The listing builds one solid part. Answer for the finished solid, in the listing's coordinates (mm). Face numbers are marked on the shaded views. A direction names the side the tool comes from. Round coordinates to 2 decimals unless told otherwise and drop trailing zeros. Loops run counter-clockwise (first coordinate to the right, second up) from the corner with the lowest first, then second, coordinate; pieces in that order, holes last. Notation, with made-up numbers: M 56.25,82 L 61.25,82 A35 cw 61.25,121 Z; hole C -12,-17 d6. An arc over 180 degrees is marked long. Answer as a JSON object with one key per item and string values.
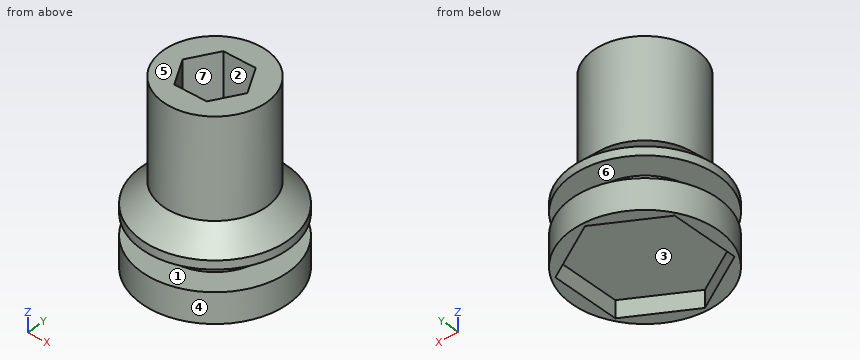
```python
from build123d import *

# Parameters (mm, degrees)
F0_R        = 8.5
F1_DEPTH    = 11
F3_DEPTH    = 2
F5_R        = 8.5
F5_R_2      = 5.5
F6_DEPTH    = 2.5
F7_R        = 6
F8_DEPTH    = 10
F9_S5_R     = 6
F9_T6_DEPTH = 14
F11_DEPTH   = 12


# Not quite as in the source:
# - a fillet or chamfer that OpenCascade refuses, or shapes differently, is made with other operations: its cross-section is extruded or revolved along the edge and cut away or added


with BuildPart() as f1:
    # F0 (on Top) → F1 (new body)
    with BuildSketch(Plane.XY):
        Circle(F0_R)
    extrude(amount=F1_DEPTH)

    # F2 (on face) → F3 (cut)
    with BuildSketch(Plane(origin=(0, 0, 0), x_dir=(1, 0, 0), z_dir=(0, 0, -1))):
        Polygon((7, 4.0414518843), (0, 8.0829037687), (-7, 4.0414518843), (-7, -4.0414518843), (0, -8.0829037687), (7, -4.0414518843), align=None)
    extrude(amount=-F3_DEPTH, mode=Mode.SUBTRACT)

    # F5 (on offset) → F6 (cut)
    with BuildSketch(Plane(origin=(0, 0, 3.5), x_dir=(1, 0, 0), z_dir=(0, 0, -1))):
        Circle(F5_R)
        Circle(F5_R_2, mode=Mode.SUBTRACT)
    extrude(amount=-F6_DEPTH, mode=Mode.SUBTRACT)

    # F7 (on face) → F8 (join)
    with BuildSketch(Plane.XY.offset(11)):
        Circle(F7_R)
    extrude(amount=F8_DEPTH)

    # F9: chamfer of 4 on 1 edges, made by hand


with BuildPart() as f9_tool2:
    # F9_s3 → F9_t4 (revolve)
    with BuildSketch(Plane.XZ):
        Polygon((8.5, 7), (4.5, 11), (8.5, 11), align=None)
    revolve(axis=Axis((0, 0, 11), (0, 0, 1)))

    # F9_s5 → F9_t6 (cut, symmetric)
    with BuildSketch(Plane.XY.offset(9)):
        Circle(F9_S5_R)
    extrude(amount=F9_T6_DEPTH, both=True, mode=Mode.SUBTRACT)


with BuildPart() as f1_1:
    add(f1.part)

    # F9_t1: cut F9_tool2
    add(f9_tool2.part, mode=Mode.SUBTRACT)

    # F10 (on face) → F11 (cut)
    with BuildSketch(Plane.XY.offset(21)):
        Polygon((3.8105117767, 0), (1.9052558883, 3.3), (-1.9052558883, 3.3), (-3.8105117767, 0), (-1.9052558883, -3.3), (1.9052558883, -3.3), align=None)
    extrude(amount=-F11_DEPTH, mode=Mode.SUBTRACT)


solid = f1_1.part
```
Item 1: Flat-ended cylindrical pins translate along their axes: P1, Ø0.6, axis at y = -2, z = 1.5, coming from the -X side; P2, Ø5, axis at y = 1.5, z = 8.5, coming from the +X side; P3, Ø1.1, axis at x = -0.5, z = 14.5, coming from the -Y side; P4, Ø1, axis at y = -2.5, z = 5, coming from the -X side. Find the tip coordinate at first contact, or state that the pin passes through.
Values follow:
{"P1": "x = -8.33", "P2": "x = 8.5", "P3": "y = -6", "P4": "x = -5.12"}
Item 2: Straight lines are drawn through the part: line 1 (Z direction, x = 1.5, y = 2.5); line 2 (Z direction, x = 5, y = 3.75); line 3 (X direction, y = 2.5, z = 11). For each, find the intervals that lie inside material, in ascending order.
Values follow:
{"line 1": "2 to 9", "line 2": "2 to 3.5, 6 to 9.25", "line 3": "-5.45 to -2.37, 2.37 to 5.45"}
Item 3: The part is cut by section B-B (z = 1.5). Give the vertices of the cut face in (x, y), then the cut area to 3 significant figures.
Values follow:
{"outline": "C 0,0 d17; hole M -7,-4.04 L 0,-8.08 L 7,-4.04 L 7,4.04 L 0,8.08 L -7,4.04 Z", "area": "57.2 mm^2"}
Item 4: The part is cut by section A-A (z = 19.75). Give the vertices of the cut face in (x, y).
Values follow:
{"outline": "C 0,0 d12; hole M -3.81,0 L -1.91,-3.3 L 1.91,-3.3 L 3.81,0 L 1.91,3.3 L -1.91,3.3 Z"}
Item 5: Determine the mould class of the marked faces 5, 6 and 7 for opening direction Z: released by +Z, released by -Z, zero draft, split by the parting line, or undercut.
Values follow:
{"face 5": "released by +Z", "face 6": "undercut", "face 7": "zero draft"}
Item 6: Which of the six approach directions +Z, -Z, +X, -X, +Y, -Y give full straight-line access (tool end or side, diameter ignored) to the marked faces 1, 2, 3 and 4?
Values follow:
{"face 1": "none", "face 2": "+Z", "face 3": "-Z", "face 4": "+Z, -Z"}
